```python
from build123d import *

# Parameters (mm, degrees)
PAD_DEPTH    = 5
POCKET_DEPTH = 3.2


with BuildPart() as part:
    # Sketch → Pad (new body)
    with BuildSketch(Plane.XY):
        with BuildLine():
            ThreePointArc((-50, -40), (-60, -50), (-50, -60))
            Line((-50, -60), (50, -60))
            ThreePointArc((50, -60), (60, -50), (50, -40))
            Line((20, -40), (50, -40))
            ThreePointArc((10, -30), (12.928932, -37.071068), (20, -40))
            Line((10, 30), (10, -30))
            ThreePointArc((20, 40), (12.928932, 37.071068), (10, 30))
            Line((50, 40), (20, 40))
            ThreePointArc((50, 40), (60, 50), (50, 60))
            Line((-50, 60), (50, 60))
            ThreePointArc((-50, 60), (-60, 50), (-50, 40))
            Line((-50, 40), (-20, 40))
            ThreePointArc((-10, 30), (-12.928932, 37.071068), (-20, 40))
            Line((-10, 30), (-10, -30))
            ThreePointArc((-20, -40), (-12.928932, -37.071068), (-10, -30))
            Line((-20, -40), (-50, -40))
        make_face()
        with BuildLine():
            ThreePointArc((-50, -48.3), (-51.7, -50), (-50, -51.7))
            Line((-50, -51.7), (-13, -51.7))
            ThreePointArc((-13, -51.7), (-11.3, -50), (-13, -48.3))
            Line((-50, -48.3), (-13, -48.3))
        make_face(mode=Mode.SUBTRACT)
        with BuildLine():
            ThreePointArc((50, -51.7), (51.7, -50), (50, -48.3))
            Line((50, -48.3), (13, -48.3))
            ThreePointArc((13, -48.3), (11.3, -50), (13, -51.7))
            Line((50, -51.7), (13, -51.7))
        make_face(mode=Mode.SUBTRACT)
        with BuildLine():
            ThreePointArc((-50, 51.7), (-51.7, 50), (-50, 48.3))
            Line((-50, 48.3), (-13, 48.3))
            ThreePointArc((-13, 48.3), (-11.3, 50), (-13, 51.7))
            Line((-50, 51.7), (-13, 51.7))
        make_face(mode=Mode.SUBTRACT)
        with BuildLine():
            ThreePointArc((50, 48.3), (51.7, 50), (50, 51.7))
            Line((50, 51.7), (13, 51.7))
            ThreePointArc((13, 51.7), (11.3, 50), (13, 48.3))
            Line((50, 48.3), (13, 48.3))
        make_face(mode=Mode.SUBTRACT)
    extrude(amount=PAD_DEPTH)

    # Sketch001 → Pocket (cut)
    with BuildSketch(Plane.XY):
        with BuildLine():
            ThreePointArc((-13, -53.4), (-9.6, -50), (-13, -46.6))
            Line((-13, -46.6), (-50, -46.6))
            ThreePointArc((-50, -46.6), (-53.4, -50), (-50, -53.4))
            Line((-13, -53.4), (-50, -53.4))
        make_face()
        with BuildLine():
            ThreePointArc((13, -46.6), (9.6, -50), (13, -53.4))
            Line((13, -53.4), (50, -53.4))
            ThreePointArc((50, -53.4), (53.4, -50), (50, -46.6))
            Line((13, -46.6), (50, -46.6))
        make_face()
        with BuildLine():
            ThreePointArc((-13, 46.6), (-9.6, 50), (-13, 53.4))
            Line((-13, 53.4), (-50, 53.4))
            ThreePointArc((-50, 53.4), (-53.4, 50), (-50, 46.6))
            Line((-13, 46.6), (-50, 46.6))
        make_face()
        with BuildLine():
            ThreePointArc((13, 53.4), (9.6, 50), (13, 46.6))
            Line((13, 46.6), (50, 46.6))
            ThreePointArc((50, 46.6), (53.4, 50), (50, 53.4))
            Line((13, 53.4), (50, 53.4))
        make_face()
    extrude(amount=POCKET_DEPTH, mode=Mode.SUBTRACT)


solid = part.part
```
Input: part model. Units: mm. Frame: model coordinates. A direction names the side the tool comes from. Round coordinates to 2 decimals unless told otherwise and drop trailing zeros. Order: outer loops, then holes, each group sorted by start corner. A loop starts at its lowest first (then second) coordinate and runs counter-clockwise, first axis right, second up. Notation, with made-up numbers: (-8.75, 81) - (9.25, 81) arc R21 cw to (9.25, 107) - close; hole circle Ø8 at (-26, 55.25). An arc over 180 degrees is marked (long way). One line per question, with ' | ' between items. Start each with the question number.
1) Cut plane C-C, the plane z = 1.95. Give the number of separate pieces and of enclosed holes in the cut face, then the cut area to 3 significant figures.
2) Cut plane D-D, the plane x = 18. Return the cut outline in (y, z), then the cut area to 3 significant figures.
3) Contact query for flat-ended pins moving along their axis: P1, Ø7.5, axis at x = -40.5, y = 51, coming from the -Z side; P2, Ø3, axis at y = -44, z = 1.5, coming from the +X side; P3, Ø2, axis at y = -42, z = 1, coming from the +X side; P4, Ø1, axis at y = 42, z = 0.5, coming from the -X side. Output: stop coordinate, or through.
4) Pull-direction query (X, two-part tool) for faces 1 (the flat face through (-1, -60, 2)), 2 (the cylindrical face through (-12.85, 36.99, 2.46)), 3 (the flat face through (31, 48, 3.2)); classes: +X half, -X half, draft (parallel to the pull), parting line (faces both ways), or undercut.
5) Set-up query: faces 4 (the flat face through (0, 5, 0)), 5 (the flat face through (31, -52, 3.2)), 6 (the flat face through (-35, -40, 2)). Return all of +Z, -Z, +X, -X, +Y, -Y with unobstructed straight access to the full face (end or side cutting, diameter ignored); none if empty.
6) Cut plane A-A, the plane x = 44.5. Return the cut outline in (y, z), then the cut area to 3 significant figures.
7) Ray query, probe 1 along Y at (x, z) = (-30, 0.55); probe 2 along Y at (x, z) = (35, 3.35); probe 3 along X at (y, z) = (-53, 3.1). Return the intervals inside material, ascending.
8) Cut plane B-B, the plane y = -50. Return the cut outline in (x, z), then the cut area to 3 significant figures.
Worked out:
1) separate pieces: 1 | enclosed holes: 4 | area: 5,160 mm^2
2) outline: (-60, 0) - (-53.4, 0) - (-53.4, 3.2) - (-51.7, 3.2) - (-51.7, 5) - (-60, 5) - close; (-48.3, 3.2) - (-46.6, 3.2) - (-46.6, 0) - (-39.8, 0) - (-39.8, 5) - (-48.3, 5) - close; (39.8, 0) - (46.6, 0) - (46.6, 3.2) - (48.3, 3.2) - (48.3, 5) - (39.8, 5) - close; (51.7, 3.2) - (53.4, 3.2) - (53.4, 0) - (60, 0) - (60, 5) - (51.7, 5) - close | area: 146 mm^2
3) P1: stops at z = 0 | P2: stops at x = 58.93 | P3: stops at x = 57.14 | P4: stops at x = -56.61
4) face 1: draft | face 2: -X half | face 3: undercut
5) face 4: -Z, +X, -X, +Y, -Y | face 5: -Z | face 6: +Z, -Z, -X
6) outline: (-60, 0) - (-53.4, 0) - (-53.4, 3.2) - (-51.7, 3.2) - (-51.7, 5) - (-60, 5) - close; (-48.3, 3.2) - (-46.6, 3.2) - (-46.6, 0) - (-40, 0) - (-40, 5) - (-48.3, 5) - close; (40, 0) - (46.6, 0) - (46.6, 3.2) - (48.3, 3.2) - (48.3, 5) - (40, 5) - close; (51.7, 3.2) - (53.4, 3.2) - (53.4, 0) - (60, 0) - (60, 5) - (51.7, 5) - close | area: 144 mm^2
7) probe 1: y = -60 to -53.4, -46.6 to -40, 40 to 46.6, 53.4 to 60 | probe 2: y = -60 to -51.7, -48.3 to -40, 40 to 48.3, 51.7 to 60 | probe 3: x = -59.54 to -51.6, -11.4 to 11.4, 51.6 to 59.54
8) outline: (-60, 0) - (-53.4, 0) - (-53.4, 3.2) - (-51.7, 3.2) - (-51.7, 5) - (-60, 5) - close; (-11.3, 3.2) - (-9.6, 3.2) - (-9.6, 0) - (9.6, 0) - (9.6, 3.2) - (11.3, 3.2) - (11.3, 5) - (-11.3, 5) - close; (51.7, 3.2) - (53.4, 3.2) - (53.4, 0) - (60, 0) - (60, 5) - (51.7, 5) - close | area: 174 mm^2
